Part model, mm, in its own coordinate system. Face numbers are marked on the shaded views. Round coordinates to 2 decimals unless told otherwise and drop trailing zeros. Loops run counter-clockwise (first coordinate to the right, second up) from the corner with the lowest first, then second, coordinate; pieces in that order, holes last.
(1) Probe probe 1 along X at (y, z) = (0.9, 0); probe 2 along X at (y, z) = (29.5, 0); probe 3 along Y at (x, z) = (4, -13). List the from-to ranges inside material, lowest first.
(2) Cut at A-A on x = 0. List the corners of the cut face in (y, z), then the cut area to 3 significant figures.
(3) Cut at B-B on z = 0. List the corners of the cut face in (x, y), then the cut area to 3 significant figures.
(4) Cut at C-C on y = 48.5. List the corners of the cut face in (x, z), then the cut area to 3 significant figures.
(5) Mould opens along Z. For the marked faces 1, 2 and 3 say: +Z half, -Z half, draft (parallel to the pull), parting line (faces both ways), or undercut.
(6) Flat gauge pins, fed straight in: pin 1 (12 mm diameter, centred on x = 3, y = 46, fed in from -Z); pin 2 (4 mm diameter, centred on x = -10, z = 0, fed in from +Y); pin 3 (4 mm diameter, centred on x = 6, y = 12, fed in from +Z); pin 4 (1.5 mm diameter, centred on x = 3.5, z = -8.5, fed in from -Y). Where does each tip first touch, or does it go through?
(7) Cut at D-D on x = -10. List the corners of the cut face in (y, z).
from build123d import *

# Parameters (mm, degrees)
SKETCH_1_R               = 5
SKETCH_1_R_2             = 3
EXTRUDE_2_DEPTH          = 60
SKETCH_2_R               = 15
SKETCH_2_R_2             = 5
EXTRUDE_3_DEPTH          = 3
HOLE_WIZARD_1_AT_2_COUNT = 2
HOLE_WIZARD_1_AT_2_PITCH = 14.142135624
HOLE_WIZARD_1_AT_3_COUNT = 2
HOLE_WIZARD_1_AT_3_PITCH = 20
HOLE_WIZARD_1_AT_4_COUNT = 2
HOLE_WIZARD_1_AT_4_PITCH = 14.142135624


with BuildPart() as part:
    # 草图1 → 凸台-拉伸2 (new body)
    with BuildSketch(Plane(origin=(0, 0, 0), x_dir=(1, 0, 0), z_dir=(0, 1, 0))):
        with Locations(Location((0, 0, 0), (0, 0, 270))):
            Circle(SKETCH_1_R)
        with Locations(Location((0, 0, 0), (0, 0, 270))):
            Circle(SKETCH_1_R_2, mode=Mode.SUBTRACT)
    extrude(amount=EXTRUDE_2_DEPTH)

    # 草图2 → 凸台-拉伸3 (add)
    with BuildSketch(Plane(origin=(0, 0, 0), x_dir=(1, 0, 0), z_dir=(0, 1, 0))):
        with Locations(Location((0, 0, 0), (0, 0, 270))):
            Circle(SKETCH_2_R)
        with Locations(Location((0, 0, 0), (0, 0, 270))):
            Circle(SKETCH_2_R_2, mode=Mode.SUBTRACT)
    extrude(amount=EXTRUDE_3_DEPTH)

    # 草图4 → 打孔尺寸(%根据)开槽沉头木螺钉的类型1 (revolve, cut)
    with BuildSketch(Plane(origin=(-10, 3, 0), x_dir=(0, 0, 1), z_dir=(1, 0, 0))):
        Polygon((0, 0), (0, 3), (1.7, 3), (1.7, 1.6), (3.3, 0), align=None)
    hole_wizard_1 = revolve(axis=Axis((-10, 9.35, 0), (0, -1, 0)), mode=Mode.SUBTRACT)

    # 打孔尺寸(%根据)开槽沉头木螺钉的类型1 at 2: 打孔尺寸(%根据)开槽沉头木螺钉的类型1 ×2
    with Locations(*[Vector(0.7071067811865476, 0, 0.7071067811865476) * (i * HOLE_WIZARD_1_AT_2_PITCH) for i in range(1, HOLE_WIZARD_1_AT_2_COUNT)]):
        add(hole_wizard_1, mode=Mode.SUBTRACT)

    # 打孔尺寸(%根据)开槽沉头木螺钉的类型1 at 3: 打孔尺寸(%根据)开槽沉头木螺钉的类型1 ×2
    with Locations(*[(i * HOLE_WIZARD_1_AT_3_PITCH, 0, 0) for i in range(1, HOLE_WIZARD_1_AT_3_COUNT)]):
        add(hole_wizard_1, mode=Mode.SUBTRACT)

    # 打孔尺寸(%根据)开槽沉头木螺钉的类型1 at 4: 打孔尺寸(%根据)开槽沉头木螺钉的类型1 ×2
    with Locations(*[Vector(0.7071067811865476, 0, -0.7071067811865476) * (i * HOLE_WIZARD_1_AT_4_PITCH) for i in range(1, HOLE_WIZARD_1_AT_4_COUNT)]):
        add(hole_wizard_1, mode=Mode.SUBTRACT)


solid = part.part
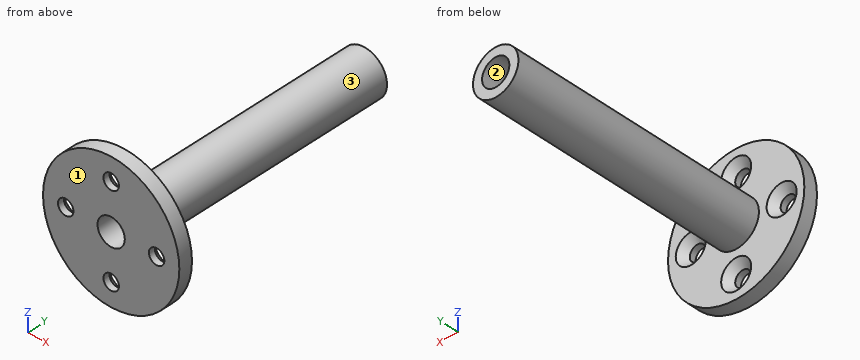
Final values:
1. probe 1: x = -15 to -11.7, -8.3 to -3, 3 to 8.3, 11.7 to 15
1. probe 2: x = -5 to -3, 3 to 5
1. probe 3: y = 0 to 3
2. outline: (0, -15) - (3, -15) - (3, -13.3) - (1.4, -11.7) - (0, -11.7) - close; (0, -8.3) - (1.4, -8.3) - (3, -6.7) - (3, -5) - (60, -5) - (60, -3) - (0, -3) - close; (0, 3) - (60, 3) - (60, 5) - (3, 5) - (3, 6.7) - (1.4, 8.3) - (0, 8.3) - close; (0, 11.7) - (1.4, 11.7) - (3, 13.3) - (3, 15) - (0, 15) - close
2. area: 274 mm2
3. outline: (-15, 0) - (-11.7, 0) - (-11.7, 1.4) - (-13.3, 3) - (-15, 3) - close; (-8.3, 0) - (-3, 0) - (-3, 60) - (-5, 60) - (-5, 3) - (-6.7, 3) - (-8.3, 1.4) - close; (3, 0) - (8.3, 0) - (8.3, 1.4) - (6.7, 3) - (5, 3) - (5, 60) - (3, 60) - close; (11.7, 0) - (15, 0) - (15, 3) - (13.3, 3) - (11.7, 1.4) - close
3. area: 274 mm2
4. outline: circle Ø10 at (0, 0); hole circle Ø6 at (0, 0)
4. area: 50.3 mm2
5. face 1: draft
5. face 2: undercut
5. face 3: parting line
6. pin 1: stops at z = -5
6. pin 2: stops at y = 1.7
6. pin 3: stops at z = 3
6. pin 4: stops at y = 0
7. outline: (0, -11.18) - (3, -11.18) - (3, -3.3) - (1.4, -1.7) - (0, -1.7) - close; (0, 1.7) - (1.4, 1.7) - (3, 3.3) - (3, 11.18) - (0, 11.18) - close
